Could you check a few things on this drawing? It's one solid part, dimensions in mm from its lowest x, y, z. Give positions to 0.01 mm unless a question says otherwise; leave off trailing zeros. Loops run counter-clockwise (first coordinate to the right, second up) from the corner with the lowest first, then second, coordinate; pieces in that order, holes last. Notation, with made-up numbers: (23.5, 71) - (70.5, 71) arc R23 cw to (70.5, 89) - close; hole circle Ø3 at (-4.5, -32). An arc over 180 degrees is marked (long way). Use a Markdown table: item, result.
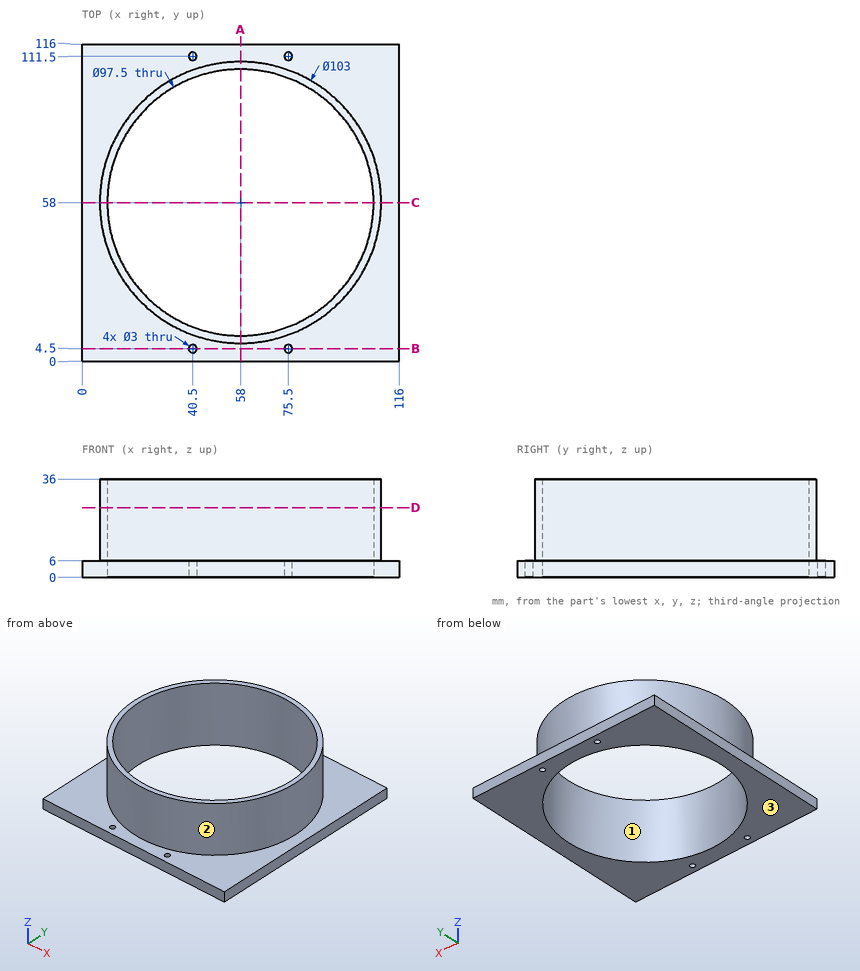
(1) Will these pins go through, and if not, where does the flat tip stop? pin 1 (5 mm diameter, centred on x = 81, z = 10.5, fed in from -Y); pin 2 (5 mm diameter, centred on x = 40.5, y = 111.5, fed in from +Z); pin 3 (1 mm diameter, centred on x = 71, z = 19.5, fed in from -Y).
A:
| item | result |
|---|---|
| pin 1 | y = 10.76 |
| pin 2 | z = 6 |
| pin 3 | y = 8.04 |
(2) If I drill on line 1 (X direction, y = 4.5, z = 3.9); line 2 (X direction, y = 4, z = 1); line 3 (Y direction, x = 75.5, z = 4.2), over which ranges is the centre line in solid material (lowest first)?
A:
| item | result |
|---|---|
| line 1 | 0 to 39, 42 to 74, 77 to 116 |
| line 2 | 0 to 39.09, 41.91 to 74.09, 76.91 to 116 |
| line 3 | 0 to 3, 6 to 12.5, 103.5 to 110, 113 to 116 |
(3) Suppose I cut it at B-B on y = 4.5. Write out the boundary of the cut face in (x, z).
A:
| item | result |
|---|---|
| outline | (0, 0) - (39, 0) - (39, 6) - (0, 6) - close; (42, 0) - (74, 0) - (74, 6) - (42, 6) - close; (77, 0) - (116, 0) - (116, 6) - (77, 6) - close |
(4) Suppose I cut it at D-D on z = 25.5. Write out the boundary of the cut face in (x, y), plus the area to 3 significant figures.
A:
| item | result |
|---|---|
| outline | circle Ø103 at (58, 58); hole circle Ø97.5 at (58, 58) |
| area | 866 mm2 |
(5) Suppose I cut it at A-A on x = 58. Write out the boundary of the cut face in (y, z), plus the area to 3 significant figures.
A:
| item | result |
|---|---|
| outline | (0, 0) - (9.25, 0) - (9.25, 36) - (6.5, 36) - (6.5, 6) - (0, 6) - close; (106.75, 0) - (116, 0) - (116, 6) - (109.5, 6) - (109.5, 36) - (106.75, 36) - close |
| area | 276 mm2 |
(6) We'd pull the mould along Y, two halves only. Please class the marked faces 1, 2 and 3: pulls with the +Y half, pulls with the -Y half, needs draft (parallel to the pull), parting line crosses it, or undercut.
A:
| item | result |
|---|---|
| face 1 | undercut |
| face 2 | parting line crosses it |
| face 3 | needs draft |
